Here's the drawing with two shaded views (mm, measured from the low corner). I have some questions. A direction names the side the tool comes from. Give positions to 0.01 mm unless a question says otherwise; leave off trailing zeros. Write each loop counter-clockwise with the first axis right and the second up, starting at its lowest first coordinate (ties: lowest second). Pieces come first, ordered by that corner, then holes.
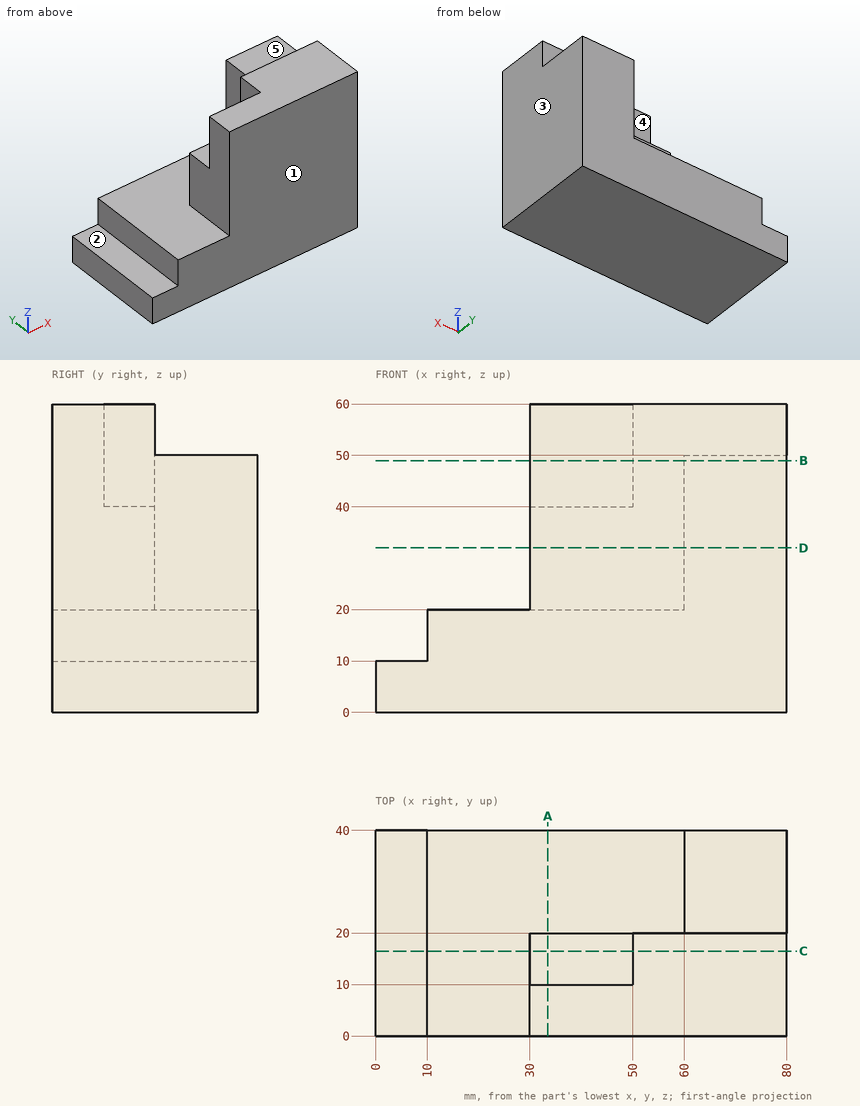
(1) Imagine slicing it at D-D, the plane z = 32. Write out the boundary of the cut face in (x, y).
Returned:
outline: (30, 0) - (80, 0) - (80, 40) - (60, 40) - (60, 20) - (30, 20) - close
(2) Imagine slicing it at B-B, the plane z = 49. Write out the boundary of the cut face in (x, y), plus the area to 3 significant figures.
Returned:
outline: (30, 0) - (80, 0) - (80, 40) - (60, 40) - (60, 20) - (50, 20) - (50, 10) - (30, 10) - close
area: 1,200 mm2
(3) If I drill on L1, parallel to X at y = 6, z = 22.5; L2, parallel to Y at x = 57.5, z = 43; L3, parallel to X at y = 4, z = 18.5, over which ranges is the centre line in solid material (lowest first)?
Returned:
L1: x = 30 to 80
L2: y = 0 to 20
L3: x = 10 to 80
(4) Imagine slicing it at C-C, the plane y = 16.5. Write out the boundary of the cut face in (x, z).
Returned:
outline: (0, 0) - (80, 0) - (80, 60) - (50, 60) - (50, 40) - (30, 40) - (30, 20) - (10, 20) - (10, 10) - (0, 10) - close
(5) For the marked faces 1, 2, 3, 4 and 5, which set-ups out of +Z, -Z, +X, -X, +Y, -Y let a thin tool reach every point of the face, with its end or its side?
Returned:
face 1: +Z, -Z, +X, -X, -Y
face 2: +Z, -X, +Y, -Y
face 3: +Z, -Z, +X, +Y, -Y
face 4: +Z, -X, +Y
face 5: +Z, +X, -X, +Y
(6) Will these pins go through, and if not, where does the flat tip stop? P1, Ø16, axis at x = 38.5, z = 54, coming from the +Y side; P2, Ø11, axis at x = 7, y = 25.5, coming from the +Z side; P3, Ø8, axis at y = 16.5, z = 46.5, coming from the -X side; P4, Ø1, axis at x = 13.5, z = 9, coming from the -Y side.
Returned:
P1: stops at y = 10
P2: stops at z = 20
P3: stops at x = 50
P4: stops at y = 0
(7) Imagine slicing it at A-A, the plane x = 33.5. Write out the boundary of the cut face in (y, z).
Returned:
outline: (0, 0) - (40, 0) - (40, 20) - (20, 20) - (20, 40) - (10, 40) - (10, 60) - (0, 60) - close
